```python
from build123d import *

# Parameters (mm, degrees)
F0_W     = 400
F0_H     = 20
F1_DEPTH = 200
F4_DEPTH = 20.001
F6_DEPTH = 20.001


with BuildPart() as f1:
    # F0 (on Top) → F1 (new body)
    with BuildSketch(Plane.XY):
        with Locations((0, -10)):
            Rectangle(F0_W, F0_H)
    extrude(amount=F1_DEPTH)

    # F3 (on face) → F4 (cut, through all)
    with BuildSketch(Plane.XZ.offset(20)):
        Polygon((-200, 117.157288), (0, 200), (-200, 200), align=None)
    extrude(amount=-F4_DEPTH, mode=Mode.SUBTRACT)

    # F5 (on face) → F6 (cut, through all)
    with BuildSketch(Plane.XZ.offset(20)):
        Polygon((200, 200), (0, 200), (200, 117.157288), align=None)
    extrude(amount=-F6_DEPTH, mode=Mode.SUBTRACT)


solid = f1.part
```
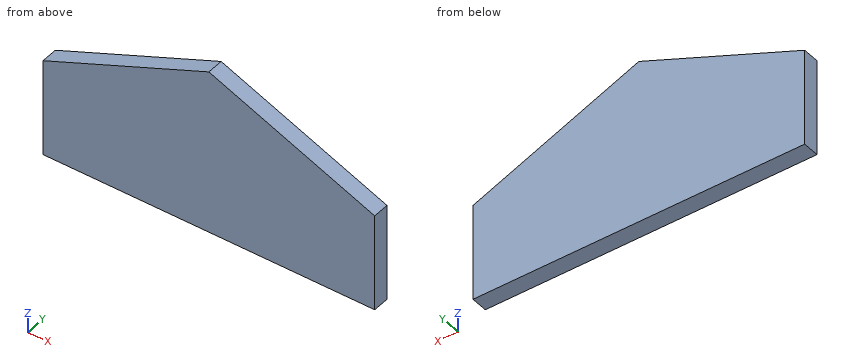
The listing builds one solid part. Answer for the finished solid, in the listing's coordinates (mm). Give positions to 0.01 mm unless a question says otherwise; leave off trailing zeros. Order: outer loops, then holes, each group sorted by start corner. A loop starts at its lowest first (then second) coordinate and runs counter-clockwise, first axis right, second up. Notation, with made-up numbers: (41, -16.5) -> (52, -16.5) arc R24 ccw to (52, 16.5) -> close; hole circle Ø7 at (78.5, 63.5). An arc over 180 degrees is marked (long way). One line per item, written item: value.
1) Find section A-A, the plane y = -9.75. Determine the outline of the cut face in (x, z).
Reported:
outline: (-200, 0) -> (200, 0) -> (200, 117.16) -> (0, 200) -> (-200, 117.16) -> close
2) Find section B-B, the plane z = 122. Determine the outline of the cut face in (x, y).
Reported:
outline: (-188.31, -20) -> (188.31, -20) -> (188.31, 0) -> (-188.31, 0) -> close
3) Find section C-C, the plane x = -22. Determine the outline of the cut face in (y, z), plus the area to 3 significant figures.
Reported:
outline: (-20, 0) -> (0, 0) -> (0, 190.89) -> (-20, 190.89) -> close
area: 3,820 mm^2
4) Find the intervals of material crossed by line 1 (Z direction, x = -161, y = -1.25); line 2 (Z direction, x = -117.5, y = -18); line 3 (X direction, y = -14, z = 144), in increasing order.
Reported:
line 1: z = 0 to 133.31
line 2: z = 0 to 151.33
line 3: x = -135.2 to 135.2
5) Flat-ended cylindrical pins translate along their axes: P1, Ø1, axis at y = -9.5, z = 120, coming from the +X side; P2, Ø1.5, axis at x = 77.5, y = -14, coming from the +Z side. Find the tip coordinate at first contact, or state that the pin passes through.
Reported:
P1: stops at x = 194.34
P2: stops at z = 168.21
